```python
from build123d import *

# Parameters (mm, degrees)
SKETCH5_R                 = 2
BOSS_EXTRUDE3_DEPTH       = 6
CHAMFER1_SIZE             = 0.5
M3X0_5_TAPPED_HOLE2_D     = 2.5
M3X0_5_TAPPED_HOLE2_DEPTH = 10
M3X0_5_TAPPED_HOLE2_TIP   = 0.751075774


with BuildPart() as part:
    # Sketch5 → Boss-Extrude3 (new body)
    with BuildSketch(Plane.XY):
        Polygon((-9.5, -6), (-11.5, -4), (-11.5, 4), (-9.5, 6), (11.5, 6), (11.5, -6), align=None)
        with Locations((-5.5, 0)):
            Circle(SKETCH5_R, mode=Mode.SUBTRACT)
    extrude(amount=BOSS_EXTRUDE3_DEPTH)

    # Chamfer1
    chamfer1_edges = [part.edges().sort_by_distance(p)[0] for p in [
        (-7.5, 0, 0),
        (-7.5, 0, 6),
    ]]
    chamfer(chamfer1_edges, length=CHAMFER1_SIZE)

    # M3x0.5 Tapped Hole2
    with Locations(Plane(origin=(11.5, 4, 2), x_dir=(0, 0, 1), z_dir=(1, 0, 0))):
        with Locations((0, 0), (0, 8)):
            Hole(M3X0_5_TAPPED_HOLE2_D / 2, depth=M3X0_5_TAPPED_HOLE2_DEPTH)
            with Locations((0, 0, -(M3X0_5_TAPPED_HOLE2_DEPTH + M3X0_5_TAPPED_HOLE2_TIP / 2))):  # 118° drill point
                Cone(0, M3X0_5_TAPPED_HOLE2_D / 2, M3X0_5_TAPPED_HOLE2_TIP, mode=Mode.SUBTRACT)


solid = part.part
```
Geometry check sheet. Reference: the model listing, model coordinates, mm. A direction names the side the tool comes from. Coordinates: 2 decimals unless noted, no trailing zeros. Order: outer loops, then holes, each group sorted by start corner. A loop starts at its lowest first (then second) coordinate and runs counter-clockwise, first axis right, second up. Notation, with made-up numbers: (56.5, 46.25) - (102.5, 46.25) arc R30 ccw to (102.5, 69.25) - close; hole circle Ø8 at (-21, 77). An arc over 180 degrees is marked (long way). Answer as a JSON object with one key per item and string values. Group by question number.
Item 1: Sectioned sample at B-B, the plane z = 5.1. Record the cut outline in (x, y), and give its area (3 significant figures).
Item 2: Sectioned sample at C-C, the plane x = -5.5. Record the cut outline in (y, z).
Item 3: Tool access check on faces 1 (the face through (0, 0, 6)), 2 (the face through (6.43, 5.109, 1.423)). Record the directions out of +Z, -Z, +X, -X, +Y, -Y that give a thin tool (end or side, any length) a straight path to the whole face; none if there is none.
Item 4: Scan lines: probe 1 along Y at (x, z) = (5, 2); probe 2 along Z at (x, y) = (9, 4); probe 3 along Y at (x, z) = (1.75, 0.9). Record each from-to range of solid material in increasing order.
Item 5: Draft check along X on faces 3 (the face through (-7.1, -1.2, 3)), 4 (the face through (11.5, 0, 3)), 5 (the face through (6.43, -2.891, 1.423)), 6 (the face through (-10.5, 5, 3)). Enter one of: +X half, -X half, draft (parallel to the pull), parting line (faces both ways), or undercut.
Item 6: Sectioned sample at A-A, the plane y = 0. Record the cut outline in (x, z).
Item 7: Depth check by flat-ended pin: pin 1 Ø3 at (y, z) = (-4, 2) entering from +X. Enter the tip coordinate at first touch or a pass-through.
Resolved:
{
 "1": {"outline": "(-11.5, -4) - (-9.5, -6) - (11.5, -6) - (11.5, 6) - (-9.5, 6) - (-11.5, 4) - close; hole circle Ø4 at (-5.5, 0)", "area": "259 mm^2"},
 "2": {"outline": "(-6, 0) - (-2.5, 0) - (-2, 0.5) - (-2, 5.5) - (-2.5, 6) - (-6, 6) - close; (2, 0.5) - (2.5, 0) - (6, 0) - (6, 6) - (2.5, 6) - (2, 5.5) - close"},
 "3": {"face 1": "+Z, +X, -X, +Y, -Y", "face 2": "+X"},
 "4": {"probe 1": "-6 to -5.25, -2.75 to 2.75, 5.25 to 6", "probe 2": "0 to 0.75, 3.25 to 6", "probe 3": "-6 to -4.59, -3.41 to 3.41, 4.59 to 6"},
 "5": {"face 3": "undercut", "face 4": "+X half", "face 5": "draft", "face 6": "-X half"},
 "6": {"outline": "(-11.5, 0) - (-8, 0) - (-7.5, 0.5) - (-7.5, 5.5) - (-8, 6) - (-11.5, 6) - close; (-3.5, 0.5) - (-3, 0) - (11.5, 0) - (11.5, 6) - (-3, 6) - (-3.5, 5.5) - close"},
 "7": {"pin 1": "x = 11.5"}
}
